Part model, mm, in its own coordinate system. Coordinates: 2 decimals unless noted, no trailing zeros. Write each loop counter-clockwise with the first axis right and the second up, starting at its lowest first coordinate (ties: lowest second). Pieces come first, ordered by that corner, then holes. Notation, with made-up numbers: (58.25, 1.25) -> (68.25, 1.25) arc R14 cw to (68.25, 20.25) -> close; hole circle Ø7 at (58.25, 77.5). An arc over 180 degrees is marked (long way). One line per question, with ' | ' between items. Start each with the question number.
Item 1: Pin check, flat tips, straight feed: pin 1 (3 mm diameter, centred on x = -153, z = 1371, fed in from +Y); pin 2 (5 mm diameter, centred on x = -22.5, y = 55, fed in from -Z); pin 3 (4 mm diameter, centred on y = 29, z = 1249.5, fed in from -X); pin 4 (6 mm diameter, centred on x = -47.5, z = 1281, fed in from +Y). Stop position of each tip, or through.
Item 2: Probe probe 1 along X at (y, z) = (44, 936); probe 2 along X at (y, z) = (54.5, 300); probe 3 along Z at (x, y) = (-102, 14.5). List the from-to ranges inside material, lowest first. Write a range as [from, to].
Item 3: Saw through at B-B (y = 79). List the corners of the cut face in (x, z), and give its area (3 significant figures).
from build123d import *

# Parameters (mm, degrees)
F0_W     = 196.85
F0_H     = 101.6
F1_DEPTH = 2438.4
F2_R     = 50.79999
F3_R     = 4.7625
F4_DEPTH = 25.4
F5_DEPTH = 25.4


# Not quite as in the source:
# - a fillet or chamfer is up to 0.001 mm smaller than in the source, because OpenCascade refuses the exact size


with BuildPart() as f1:
    # F0 (on Top) → F1 (new body)
    with BuildSketch(Plane.XY):
        with Locations((-98.425, 50.8)):
            Rectangle(F0_W, F0_H)
    extrude(amount=F1_DEPTH)

    # F2 (radius 50.8 in the source; OpenCascade refuses exactly that, so slightly less here)
    f2_edges = [f1.edges().sort_by_distance(p)[0] for p in [
        (0, 0, 1219.2),
        (-196.85, 0, 1219.2),
        (-196.85, 101.6, 1219.2),
        (0, 101.6, 1219.2),
    ]]
    fillet(f2_edges, radius=F2_R)

    # F3 (on face) → F4 (cut)
    with BuildSketch(Plane.XZ):
        with Locations((-98.425, 1220.7875)):
            Circle(F3_R)
    extrude(amount=-F4_DEPTH, mode=Mode.SUBTRACT)

    # F3 (on face) → F5 (cut)
    with BuildSketch(Plane.XZ):
        with Locations((-98.425, 1220.7875)):
            Circle(F3_R)
    extrude(amount=-F5_DEPTH, mode=Mode.SUBTRACT)


solid = f1.part
From the geometry:
1) pin 1: y = 101.31 | pin 2: z = 0 | pin 3: x = -192.83 | pin 4: y = 101.6
2) probe 1: [-196.39, -0.46] | probe 2: [-196.72, -0.13] | probe 3: [0, 1217.64], [1223.93, 2438.4]
3) outline: (-188.3, 0) -> (-8.55, 0) -> (-8.55, 2438.4) -> (-188.3, 2438.4) -> close | area: 438,000 mm2
